Source: CAD feature listing. Evaluate the final solid. Frame: model axes, mm. A direction names the side the tool comes from. Give positions to 0.01 mm unless a question says otherwise; leave off trailing zeros. Order: outer loops, then holes, each group sorted by start corner. A loop starts at its lowest first (then second) coordinate and runs counter-clockwise, first axis right, second up. Notation, with made-up numbers: (6, -32) - (24, -32) arc R20 ccw to (24, -23) - close; hole circle Ø3 at (31, 15). An arc over 180 degrees is marked (long way). Use CSV: the item, a comma, the result in double quotes.
```python
from build123d import *

# Parameters (mm, degrees)
SKETCH1_W               = 110
SKETCH1_H               = 80
SKETCH1_R               = 1.375
BOSS_EXTRUDE1_DEPTH     = 3
SKETCH3_W               = 3
SKETCH3_H               = 80
BOSS_EXTRUDE2_DEPTH     = 45
CUT_EXTRUDE1_DEPTH      = 141.292551477
CUT_EXTRUDE1_DEPTH_BACK = 141.292551477
SKETCH4_R               = 1.5
CUT_EXTRUDE2_DEPTH      = 138.764291455
CUT_EXTRUDE2_DEPTH_BACK = 138.764291455
SKETCH5_W               = 3
SKETCH5_H               = 80


with BuildPart() as part:
    # Sketch1 → Boss-Extrude1 (new body)
    with BuildSketch(Plane(origin=(0, 0, 0), x_dir=(1, 0, 0), z_dir=(0, 1, 0))):
        with Locations((50, 37)):
            Rectangle(SKETCH1_W, SKETCH1_H)
        with Locations(Location((5, 11, 0), (0, 0, 270))):
            Circle(SKETCH1_R, mode=Mode.SUBTRACT)
        with Locations(Location((5, 69, 0), (0, 0, 270))):
            Circle(SKETCH1_R, mode=Mode.SUBTRACT)
        with Locations(Location((91, 69, 0), (0, 0, 270))):
            Circle(SKETCH1_R, mode=Mode.SUBTRACT)
        with Locations(Location((91, 11, 0), (0, 0, 270))):
            Circle(SKETCH1_R, mode=Mode.SUBTRACT)
    extrude(amount=BOSS_EXTRUDE1_DEPTH)

    # Sketch3 → Boss-Extrude2 (add)
    with BuildSketch(Plane(origin=(0, 3, 0), x_dir=(1, 0, 0), z_dir=(0, 1, 0))):
        with Locations((-3.5, 37)):
            Rectangle(SKETCH3_W, SKETCH3_H)
        with Locations((103.5, 37)):
            Rectangle(SKETCH3_W, SKETCH3_H)
    extrude(amount=BOSS_EXTRUDE2_DEPTH)

    # Sketch4 → Cut-Extrude1 (cut, two sides: drawn at the far end of the back side and taken through both)
    with BuildSketch(Plane.ZY.offset(-102).offset(-CUT_EXTRUDE1_DEPTH_BACK)):
        with Locations((-72, 42)):
            Circle(SKETCH4_R)
        with Locations((-2, 42)):
            Circle(SKETCH4_R)
    extrude(amount=CUT_EXTRUDE1_DEPTH + CUT_EXTRUDE1_DEPTH_BACK, mode=Mode.SUBTRACT)

    # Sketch5 → Cut-Extrude2 (cut, two sides: drawn at the far end of the back side and taken through both)
    with BuildSketch(Plane(origin=(0, 3, 0), x_dir=(1, 0, 0), z_dir=(0, 1, 0)).offset(-CUT_EXTRUDE2_DEPTH_BACK)):
        with Locations((-3.5, 37)):
            Rectangle(SKETCH5_W, SKETCH5_H)
    extrude(amount=CUT_EXTRUDE2_DEPTH + CUT_EXTRUDE2_DEPTH_BACK, mode=Mode.SUBTRACT)


solid = part.part
```
Item 1: First-contact query: pin 1 (3 mm diameter, centred on x = 91, z = -11, fed in from +Y); pin 2 (5 mm diameter, centred on y = 42, z = -66.5, fed in from -X). Flat tips, straight axial feed; report the tip coordinate or a pass-through.
Filled in:
pin 1,"stops at y = 3"
pin 2,"stops at x = 102"
Item 2: Section D-D on z = -30.5. Return the cut outline in (x, y), then the cut area to 3 significant figures.
Filled in:
outline,"(-2, 0) - (105, 0) - (105, 48) - (102, 48) - (102, 3) - (-2, 3) - close"
area,"456 mm2"
Item 3: Material intervals for line 1 (X direction, y = 1, z = -69) (3 decimals); line 2 (Z direction, x = 103, y = 42); line 3 (Y direction, x = 103.85, z = -2), sorted ascending. Write a range as from..to.
Filled in:
line 1,"x = -2..3.625, 6.375..89.625, 92.375..105"
line 2,"z = -77..-73.5, -70.5..-3.5, -0.5..3"
line 3,"y = 0..40.5, 43.5..48"
Item 4: Section A-A on z = -72. Return the cut outline in (x, y), then the cut area to 3 significant figures.
Filled in:
outline,"(-2, 0) - (105, 0) - (105, 40.5) - (102, 40.5) - (102, 3) - (-2, 3) - close; (102, 43.5) - (105, 43.5) - (105, 48) - (102, 48) - close"
area,"447 mm2"
Item 5: Section C-C on y = 19.5. Return the cut outline in (x, z), then the cut area to 3 significant figures.
Filled in:
outline,"(102, -77) - (105, -77) - (105, 3) - (102, 3) - close"
area,"240 mm2"
Item 6: Mould query, pull axis X, two halves, no side actions, for faces 3 (the cylindrical face through (89.66, 1.48, -11.3)), 4 (the flat face through (105, 24, -36)), 5 (the flat face through (51, 0, -38)). Classes: released by +X, released by -X, zero draft, split by the parting line, or undercut.
Filled in:
face 3,"undercut"
face 4,"released by +X"
face 5,"zero draft"
Item 7: Section B-B on x = 5. Return the cut outline in (y, z) (3 decimals), then the cut area to 4 significant figures.
Filled in:
outline,"(0, -77) - (3, -77) - (3, -70.375) - (0, -70.375) - close; (0, -67.625) - (3, -67.625) - (3, -12.375) - (0, -12.375) - close; (0, -9.625) - (3, -9.625) - (3, 3) - (0, 3) - close"
area,"223.5 mm2"
Item 8: Set-up query: faces 1 (the cylindrical face through (103.521, 40.536, -2.325)), 2 (the flat face through (102, 25, -36)). Return all of +Z, -Z, +X, -X, +Y, -Y with unobstructed straight access to the full face (end or side cutting, diameter ignored); none if empty.
Filled in:
face 1,"+X, -X"
face 2,"+Z, -Z, -X, +Y"
